Work out the finished part from the listing and answer in its coordinate system (mm). Face numbers are marked on the shaded views. A direction names the side the tool comes from. Coordinates: 2 decimals unless noted, no trailing zeros. Loops run counter-clockwise (first coordinate to the right, second up) from the corner with the lowest first, then second, coordinate; pieces in that order, holes last. Notation, with made-up numbers: (50, -27) -> (76, -27) arc R17 ccw to (76, -23) -> close; hole circle Ø6 at (48, 77.5). An arc over 180 degrees is marked (long way). One line per question, with ' | ' between items.
```python
from build123d import *

# Parameters (mm, degrees)
F5_DEPTH = 40
F6_DEPTH = 40


with BuildPart() as f5:
    # F4 (on Top) → F5 (new body)
    with BuildSketch(Plane.XY):
        Polygon((-30, 0), (-80, 0), (-80, -14.75), (-69.75, -14.75), (-69.75, -24.75), (-40.25, -24.75), (-40.25, -14.75), (-30, -14.75), align=None)
    extrude(amount=-F5_DEPTH)

    # F4 (on Top) → F6 (join)
    with BuildSketch(Plane.XY):
        Polygon((-69.75, 14.75), (-80, 14.75), (-80, 0), (-30, 0), (-30, 14.75), (-40.25, 14.75), (-40.25, 24.75), (-69.75, 24.75), align=None)
        Polygon((-30, 0), (-80, 0), (-80, -14.75), (-69.75, -14.75), (-69.75, -24.75), (-40.25, -24.75), (-40.25, -14.75), (-30, -14.75), align=None)
    extrude(amount=-F6_DEPTH)


solid = f5.part
```
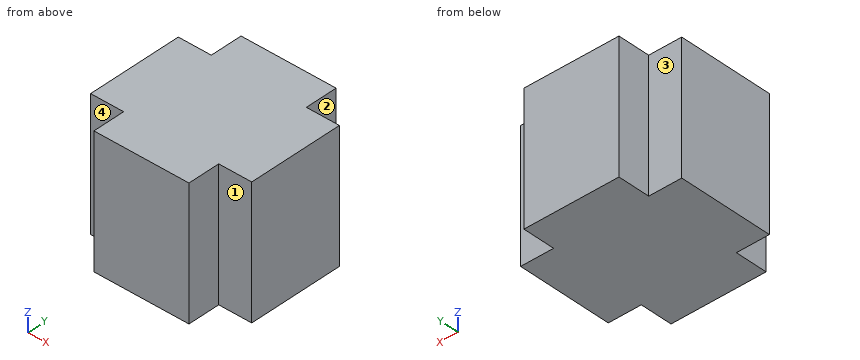
1) Flat-ended cylindrical pins translate along their axes: pin 1 (3 mm diameter, centred on y = -19, z = -29.5, fed in from +X); pin 2 (11.5 mm diameter, centred on x = -33.5, z = -18.5, fed in from -Y); pin 3 (5 mm diameter, centred on x = -73, z = -21.5, fed in from +Y); pin 4 (10 mm diameter, centred on x = -43, y = 11.5, fed in from +Z). Find the tip coordinate at first contact, or state that the pin passes through.
Check values:
pin 1: stops at x = -40.25 | pin 2: stops at y = -14.75 | pin 3: stops at y = 14.75 | pin 4: stops at z = 0
2) Find section C-C (x = -75). Write down the section's boundary in (y, z).
Check values:
outline: (-14.75, -40) -> (14.75, -40) -> (14.75, 0) -> (-14.75, 0) -> close
3) For the marked faces 1, 2, 3 and 4, determine the directions among +Z, -Z, +X, -X, +Y, -Y from which every point of the face is accessible in a straight line to the end or side of a thin tool.
Check values:
face 1: +Z, -Z, +X, -Y | face 2: +Z, -Z, +X, +Y | face 3: +Z, -Z, -X, +Y | face 4: +Z, -Z, -X, -Y
4) Find the intervals of material crossed by line 1 along Y through (x, z) = (-76.5, -10); line 2 along X through (y, z) = (19, -18), in increasing order.
Check values:
line 1: y = -14.75 to 14.75 | line 2: x = -69.75 to -40.25
5) Find section B-B (y = -15.5). Write down the section's boundary in (x, z), plus the area to 3 significant figures.
Check values:
outline: (-69.75, -40) -> (-40.25, -40) -> (-40.25, 0) -> (-69.75, 0) -> close | area: 1,180 mm^2
6) Find section A-A (z = -4.5). Write down the section's boundary in (x, y).
Check values:
outline: (-80, -14.75) -> (-69.75, -14.75) -> (-69.75, -24.75) -> (-40.25, -24.75) -> (-40.25, -14.75) -> (-30, -14.75) -> (-30, 14.75) -> (-40.25, 14.75) -> (-40.25, 24.75) -> (-69.75, 24.75) -> (-69.75, 14.75) -> (-80, 14.75) -> close
